from build123d import *

# Parameters (mm, degrees)
SKETCH_1_W          = 115
SKETCH_1_H          = 90
EXTRUDE_1_DEPTH     = 15
SKETCH_2_W          = 110
SKETCH_2_H          = 85
CUT_EXTRUDE_1_DEPTH = 13
SKETCH_4_R          = 2.5
CUT_EXTRUDE_2_DEPTH = 13
CUT_EXTRUDE_3_DEPTH = 10
EXTRUDE_2_DEPTH     = 13
SKETCH_8_W          = 23.526984817
SKETCH_8_H          = 13.315340632
SKETCH_8_W_2        = 23.473015183
SKETCH_8_H_2        = 13.660063904
SKETCH_8_H_3        = 13.684659368
EXTRUDE_4_DEPTH     = 5
FILLET_1_R          = 4
FILLET_2_R          = 4
SKETCH_9_R          = 2.5
CUT_EXTRUDE_4_DEPTH = 25


with BuildPart() as part:
    # Эскиз1 → Бобышка-Вытянуть1 (new body)
    with BuildSketch(Plane(origin=(0, 0, 0), x_dir=(1, 0, 0), z_dir=(0, 1, 0))):
        with Locations((-0.217418325, 0.217418325)):
            Rectangle(SKETCH_1_W, SKETCH_1_H)
    extrude(amount=EXTRUDE_1_DEPTH)

    # Эскиз2 → Вырез-Вытянуть1 (cut)
    with BuildSketch(Plane.XZ):
        Rectangle(SKETCH_2_W, SKETCH_2_H)
    extrude(amount=-CUT_EXTRUDE_1_DEPTH, mode=Mode.SUBTRACT)

    # Эскиз4 → Вырез-Вытянуть2 (cut)
    with BuildSketch(Plane(origin=(0, 15, 0), x_dir=(1, 0, 0), z_dir=(0, 1, 0))):
        with Locations(Location((-50.146124261, 38.945020388, 0), (0, 0, 270))):
            Circle(SKETCH_4_R)
        with Locations(Location((50.678785721, -39.961430902, 0), (0, 0, 270))):
            Circle(SKETCH_4_R)
        with Locations(Location((-50.146124261, -39.961430902, 0), (0, 0, 270))):
            Circle(SKETCH_4_R)
        with Locations(Location((50.678785721, 38.945020388, 0), (0, 0, 270))):
            Circle(SKETCH_4_R)
    extrude(amount=-CUT_EXTRUDE_2_DEPTH, mode=Mode.SUBTRACT)

    # Эскиз5 → Вырез-Вытянуть3 (cut)
    with BuildSketch(Plane(origin=(0, 15, 0), x_dir=(1, 0, 0), z_dir=(0, 1, 0))):
        Polygon((-56.190433508, 33.532758957), (-36.190433508, 33.532758957), (-36.190433508, 43.532758957), (-36.190433508, 45.217418325), (-57.717418325, 45.217418325), (-57.717418325, 33.532758957), align=None)
        Polygon((-56.190433508, -33.467241043), (-36.190433508, -33.467241043), (-36.190433508, -43.467241043), (-36.190433508, -44.782581675), (-57.717418325, -44.782581675), (-57.717418325, -33.467241043), align=None)
        Polygon((55.809566492, -33.467241043), (35.809566492, -33.467241043), (35.809566492, -43.467241043), (35.809566492, -44.782581675), (57.282581675, -44.782581675), (57.282581675, -33.467241043), align=None)
        Polygon((55.809566492, 33.532758957), (35.809566492, 33.532758957), (35.809566492, 43.532758957), (35.809566492, 45.217418325), (57.282581675, 45.217418325), (57.282581675, 33.532758957), align=None)
    extrude(amount=-CUT_EXTRUDE_3_DEPTH, mode=Mode.SUBTRACT)

    # Эскиз6 → Бобышка-Вытянуть2 (add)
    with BuildSketch(Plane.XZ.offset(-13)):
        Polygon((-55, -33.532758957), (-36.190433508, -33.532758957), (-36.190433508, -42.5), (-34.190433508, -42.5), (-34.190433508, -31.557354421), (-34.190433508, -31.532758957), (-35.500302021, -31.532758957), (-55, -31.532758957), align=None)
        Polygon((-36.190433508, 42.5), (-34.190433508, 42.5), (-34.190433508, 31.467241043), (-55, 31.467241043), (-55, 33.467241043), (-36.190433508, 33.467241043), align=None)
        Polygon((35.809566492, 42.5), (33.809566492, 42.5), (33.809566492, 31.467241043), (55, 31.467241043), (55, 33.467241043), (35.809566492, 33.467241043), align=None)
        Polygon((35.809566492, -42.5), (33.809566492, -42.5), (33.809566492, -31.557354421), (55, -31.557354421), (55, -33.532758957), (35.809566492, -33.532758957), align=None)
    extrude(amount=EXTRUDE_2_DEPTH)

    # Эскиз8 → Бобышка-Вытянуть4 (add)
    with BuildSketch(Plane.XZ):
        with Locations((-45.953925917, 38.124911359)):
            Rectangle(SKETCH_8_W, SKETCH_8_H)
        with Locations((45.546074084, 38.124911359)):
            Rectangle(SKETCH_8_W_2, SKETCH_8_H)
        with Locations((45.546074084, -38.387386373)):
            Rectangle(SKETCH_8_W_2, SKETCH_8_H_2)
        with Locations((-45.953925917, -38.375088641)):
            Rectangle(SKETCH_8_W, SKETCH_8_H_3)
    extrude(amount=-EXTRUDE_4_DEPTH)

    # Скругление1
    fillet_1_edges = [part.edges().sort_by_distance(p)[0] for p in [
        (-57.717418325, 10, 33.467241043),
        (-36.190433508, 10, 44.782581675),
        (-36.190433508, 10, -45.217418325),
        (-57.717418325, 10, -33.532758957),
        (-36.190433508, 10, 33.467241043),
        (35.809566492, 10, 33.467241043),
        (35.809566492, 10, -33.532758957),
        (-36.190433508, 10, -33.532758957),
        (57.282581675, 2.5, 44.782581675),
        (-57.717418325, 2.5, 44.782581675),
        (-57.717418325, 2.5, -45.217418325),
        (57.282581675, 2.5, -45.217418325),
        (57.282581675, 10, -33.532758957),
        (35.809566492, 10, -45.217418325),
        (35.809566492, 10, 44.782581675),
        (57.282581675, 10, 33.467241043),
    ]]
    fillet(fillet_1_edges, radius=FILLET_1_R)

    # Скругление2
    fillet_2_edges = [part.edges().sort_by_distance(p)[0] for p in [
        (-55, 6.5, -31.532758957),
        (-34.190433508, 6.5, -42.5),
        (-34.190433508, 6.5, -31.532758957),
        (-55, 6.5, 31.467241043),
        (-34.190433508, 6.5, 31.467241043),
        (-34.190433508, 6.5, 42.5),
        (33.809566492, 6.5, 42.5),
        (33.809566492, 6.5, 31.467241043),
        (55, 6.5, 31.467241043),
        (55, 6.5, -31.557354421),
        (33.809566492, 6.5, -31.557354421),
        (33.809566492, 6.5, -42.5),
    ]]
    fillet(fillet_2_edges, radius=FILLET_2_R)

    # Эскиз9 → Вырез-Вытянуть4 (cut)
    with BuildSketch(Plane(origin=(0, 15, 0), x_dir=(1, 0, 0), z_dir=(0, 1, 0))):
        with Locations(Location((-50.508936052, 39.912518498, 0), (0, 0, 270))):
            Circle(SKETCH_9_R)
        with Locations(Location((50.315973929, -38.993932792, 0), (0, 0, 270))):
            Circle(SKETCH_9_R)
        with Locations(Location((-50.508936052, -38.993932792, 0), (0, 0, 270))):
            Circle(SKETCH_9_R)
        with Locations(Location((50.315973929, 39.912518498, 0), (0, 0, 270))):
            Circle(SKETCH_9_R)
    extrude(amount=-CUT_EXTRUDE_4_DEPTH, mode=Mode.SUBTRACT)


solid = part.part
The model under review builds one solid part; all positions refer to its coordinate system, in mm. A direction names the side the tool comes from. Give positions to 0.01 mm unless a question says otherwise; leave off trailing zeros. Write each loop counter-clockwise with the first axis right and the second up, starting at its lowest first coordinate (ties: lowest second). Pieces come first, ordered by that corner, then holes.
1. Add section D-D, the plane x = -2. Write out the cut boundary in (y, z), plus the area to 3 significant figures.
2. Draft analysis for pull direction X (two halves, no side actions). For faces 5 (the cylindrical face through (56.142, 2.535, -44.015)), 6 (the cylindrical face through (-33.05, 6.591, -41.297)), 7 (the cylindrical face through (-34.988, 9.93, -44.077)), state which applies: +X half, -X half, draft (parallel to the pull), parting line (faces both ways), or undercut.
3. For P1, Ø7.5, axis at x = 48, z = 40, coming from the +Y side; P2, Ø1.5, axis at x = 32, z = -10, coming from the -Y side; P3, Ø4, axis at x = 50.32, z = -39.91, coming from the +Y side; P4, Ø1, axis at y = 8.5, z = 39, coming from the -X side, all flat-tipped, find the tip position at first contact; note any pin that passes through.
4. Wall thickness on L1, parallel to X at y = 2, z = -17.5; L2, parallel to Z at x = 18, y = 11.25; L3, parallel to X at y = 12, z = -38: over which ranges is each line inside the solid? List them lowest first.
5. Add section A-A, the plane z = 11. Write out the cut boundary in (x, y).
6. Tool access review of faces 1 (the cylindrical face through (-32.988, 6.409, 41.359)), 2 (the cylindrical face through (34.669, 9.93, -44.015)), 3 (the cylindrical face through (-56.577, 9.93, -32.33)), 4 (the flat face through (44, 5, 39)): name each direction out of +Z, -Z, +X, -X, +Y, -Y from which nothing blocks a thin tool from reaching the whole face with its end or side.
7. Add section B-B, the plane x = -42.5. Write out the cut boundary in (y, z), plus the area to 3 significant figures.
8. Add section C-C, the plane y = 2.25. Count the separate pieces of the cut face and the enclosed holes in it, plus the area to 3 significant figures.
Worked answers:
1. outline: (0, -45.22) - (15, -45.22) - (15, 44.78) - (0, 44.78) - (0, 42.5) - (13, 42.5) - (13, -42.5) - (0, -42.5) - close
1. area: 245 mm2
2. face 5: +X half
2. face 6: undercut
2. face 7: -X half
3. P1: stops at y = 5
3. P2: stops at y = 13
3. P3: passes through
3. P4: stops at x = -36.19
4. L1: x = -57.72 to -55, 55 to 57.28
4. L2: z = -45.22 to -42.5, 42.5 to 44.78
4. L3: x = -36.19 to -34.19, 33.81 to 35.81
5. outline: (-57.72, 0) - (-55, 0) - (-55, 13) - (55, 13) - (55, 0) - (57.28, 0) - (57.28, 15) - (-57.72, 15) - close
6. face 1: -Y
6. face 2: -Z, +X, +Y
6. face 3: -Z, -X, +Y
6. face 4: +Z, +X, +Y
7. outline: (0, -45.22) - (5, -45.22) - (5, -33.53) - (15, -33.53) - (15, 33.47) - (5, 33.47) - (5, 44.78) - (0, 44.78) - (0, 31.47) - (13, 31.47) - (13, -31.53) - (0, -31.53) - close
7. area: 301 mm2
8. separate pieces: 1
8. enclosed holes: 5
8. area: 1,840 mm2
